from build123d import *

# Parameters (mm, degrees)
SKETCH_1_W          = 15
SKETCH_1_H          = 15
SKETCH_1_W_2        = 13
SKETCH_1_H_2        = 13
EXTRUDE_1_DEPTH     = 230
SKETCH_2_R          = 1.5
CUT_EXTRUDE_1_DEPTH = 231.610602532


with BuildPart() as part:
    # 草图1 → 凸台-拉伸1 (new body)
    with BuildSketch(Plane(origin=(0, 0, 0), x_dir=(1, 0, 0), z_dir=(0, 1, 0))):
        Rectangle(SKETCH_1_W, SKETCH_1_H)
        Rectangle(SKETCH_1_W_2, SKETCH_1_H_2, mode=Mode.SUBTRACT)
    extrude(amount=EXTRUDE_1_DEPTH)

    # 草图2 → 切除-拉伸1 (cut, through all)
    with BuildSketch(Plane(origin=(7.5, 0, 0), x_dir=(0, 0, -1), z_dir=(1, 0, 0))):
        with Locations((0, 160)):
            Circle(SKETCH_2_R)
        with Locations((0, 138)):
            Circle(SKETCH_2_R)
        with Locations((0, 182)):
            Circle(SKETCH_2_R)
        with Locations(Location((0, 48, 0), (0, 0, 180))):
            Circle(SKETCH_2_R)
        with Locations(Location((0, 92, 0), (0, 0, 180))):
            Circle(SKETCH_2_R)
        with Locations(Location((0, 70, 0), (0, 0, 180))):
            Circle(SKETCH_2_R)
    extrude(amount=-CUT_EXTRUDE_1_DEPTH, mode=Mode.SUBTRACT)


solid = part.part
For this review, take the finished solid that the model builds, in its own axes (mm). A direction names the side the tool comes from. Coordinates: 2 decimals unless noted, no trailing zeros. Order: outer loops, then holes, each group sorted by start corner. A loop starts at its lowest first (then second) coordinate and runs counter-clockwise, first axis right, second up. Notation, with made-up numbers: (-20, 9) -> (25, 9) arc R14 cw to (25, 15) -> close; hole circle Ø4 at (22, 80.25). An arc over 180 degrees is marked (long way). Return JSON: item names as keys, results as strings.
1. The part is to be moulded in two halves that separate along X. For faces 1 (the flat face through (-6.5, 113, 0)), 2 (the flat face through (0, 113, 6.5)), 3 (the flat face through (-7, 0, 0)), 4 (the flat face through (7.5, 113, 0)), say which applies: +X half, -X half, draft (parallel to the pull), parting line (faces both ways), or undercut.
Answer block:
{"face 1": "undercut", "face 2": "undercut", "face 3": "draft", "face 4": "+X half"}
2. We need section B-B on y = 31.5. Write out the cut boundary in (x, z).
Answer block:
{"outline": "(-7.5, -7.5) -> (7.5, -7.5) -> (7.5, 7.5) -> (-7.5, 7.5) -> close; hole (-6.5, -6.5) -> (6.5, -6.5) -> (6.5, 6.5) -> (-6.5, 6.5) -> close"}
3. We need section A-A on x = -2.75. Write out the cut boundary in (y, z), and give its area (3 significant figures).
Answer block:
{"outline": "(0, -7.5) -> (230, -7.5) -> (230, -6.5) -> (0, -6.5) -> close; (0, 6.5) -> (230, 6.5) -> (230, 7.5) -> (0, 7.5) -> close", "area": "460 mm²"}
4. Machinability: for faces 5 (the flat face through (0, 113, 7.5)), 6 (the flat face through (6.5, 113, 0)), which of the approach directions +Z, -Z, +X, -X, +Y, -Y give a long, thin tool a straight path to every point of the face, cutting with its end or side? Answer none if there is none.
Answer block:
{"face 5": "+Z, +X, -X, +Y, -Y", "face 6": "+Y, -Y"}
5. For line 1 (Z direction, x = -6.9, y = 70); line 2 (X direction, y = 19, z = -2.5), list the stretches that pass through material, from the lowest coordinate up. Write a range as from..to.
Answer block:
{"line 1": "-7.5..-1.5, 1.5..7.5", "line 2": "-7.5..-6.5, 6.5..7.5"}
